from build123d import *

# Parameters (mm, degrees)
EXTRUDE_1_DEPTH     = 38
SKETCH_2_R          = 2.75
CUT_EXTRUDE_1_DEPTH = 21
CUT_EXTRUDE_2_DEPTH = 21


with BuildPart() as part:
    # 草图1 → 凸台-拉伸1 (new body)
    with BuildSketch(Plane(origin=(0, 0, 0), x_dir=(0, 0, -1), z_dir=(1, 0, 0))):
        Polygon((0, 0), (20, 0), (20, 3), (3, 3), (3, 20), (0, 20), align=None)
    extrude(amount=EXTRUDE_1_DEPTH)

    # 草图2 → 切除-拉伸1 (cut, through all)
    with BuildSketch(Plane.XY):
        with Locations((9, 10)):
            Circle(SKETCH_2_R)
        with Locations((29, 10)):
            Circle(SKETCH_2_R)
    extrude(amount=-CUT_EXTRUDE_1_DEPTH, mode=Mode.SUBTRACT)

    # 草图3 → 切除-拉伸2 (cut, through all)
    with BuildSketch(Plane.XZ):
        with BuildLine():
            Line((6.25, -13.5), (6.25, -6.5))
            ThreePointArc((6.25, -6.5), (9, -3.75), (11.75, -6.5))
            Line((11.75, -6.5), (11.75, -13.5))
            ThreePointArc((11.75, -13.5), (9, -16.25), (6.25, -13.5))
        make_face()
        with BuildLine():
            Line((26.25, -13.5), (26.25, -6.5))
            ThreePointArc((26.25, -6.5), (29, -3.75), (31.75, -6.5))
            Line((31.75, -6.5), (31.75, -13.5))
            ThreePointArc((31.75, -13.5), (29, -16.25), (26.25, -13.5))
        make_face()
    extrude(amount=-CUT_EXTRUDE_2_DEPTH, mode=Mode.SUBTRACT)


solid = part.part
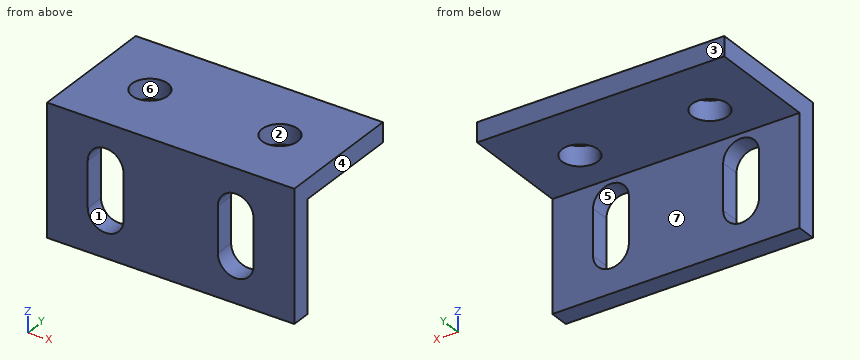
The listing builds one solid part. Answer for the finished solid, in the listing's coordinates (mm). Face numbers are marked on the shaded views. A direction names the side the tool comes from. Give positions to 0.01 mm unless a question says otherwise; leave off trailing zeros. Order: outer loops, then holes, each group sorted by start corner. A loop starts at its lowest first (then second) coordinate and runs counter-clockwise, first axis right, second up. Notation, with made-up numbers: (4, 23) - (42, 23) arc R13 ccw to (42, 43) - close; hole circle Ø7 at (2.5, -3.5). An arc over 180 degrees is marked (long way). Answer as CSV lines item,"result".
Q1. A cutting plane is placed at A-A, the plane y = 10. Determine the outline of the cut face in (x, z).
Answer key:
outline,"(0, -3) - (6.25, -3) - (6.25, 0) - (0, 0) - close; (11.75, -3) - (26.25, -3) - (26.25, 0) - (11.75, 0) - close; (31.75, -3) - (38, -3) - (38, 0) - (31.75, 0) - close"
Q2. Determine the mould class of the marked faces 1, 2, 3 and 4 for opening direction X: pulls with the +X half, pulls with the -X half, needs draft (parallel to the pull), parting line crosses it, or undercut.
Answer key:
face 1,"undercut"
face 2,"undercut"
face 3,"needs draft"
face 4,"pulls with the +X half"
Q3. Each of these flat-tipped pins is pushed along its axis until it touches: pin 1 Ø1 at (x, y) = (28.5, 14.5) entering from -Z; pin 2 Ø10 at (x, z) = (25, -8.5) entering from +Y. Where does it stop, or does it pass through?
Answer key:
pin 1,"stops at z = -3"
pin 2,"stops at y = 3"
Q4. Which of the six approach directions +Z, -Z, +X, -X, +Y, -Y give full straight-line access (tool end or side, diameter ignored) to the marked faces 5, 6 and 7?
Answer key:
face 5,"+Y, -Y"
face 6,"+Z, -Z"
face 7,"-Z, +X, -X, +Y"
Q5. A cutting plane is placed at C-C, the plane z = -5.75. Determine the outline of the cut face in (x, y), and give its area (3 significant figures).
Answer key:
outline,"(0, 0) - (6.35, 0) - (6.35, 3) - (0, 3) - close; (11.65, 0) - (26.35, 0) - (26.35, 3) - (11.65, 3) - close; (31.65, 0) - (38, 0) - (38, 3) - (31.65, 3) - close"
area,"82.3 mm^2"
Q6. A cutting plane is placed at D-D, the plane z = -17.5. Determine the outline of the cut face in (x, y), and give its area (3 significant figures).
Answer key:
outline,"(0, 0) - (38, 0) - (38, 3) - (0, 3) - close"
area,"114 mm^2"
Q7. A cutting plane is placed at B-B, the plane x = 29. Determine the outline of the cut face in (y, z), and give its area (3 significant figures).
Answer key:
outline,"(0, -20) - (3, -20) - (3, -16.25) - (0, -16.25) - close; (0, -3.75) - (3, -3.75) - (3, -3) - (7.25, -3) - (7.25, 0) - (0, 0) - close; (12.75, -3) - (20, -3) - (20, 0) - (12.75, 0) - close"
area,"57.0 mm^2"
Q8. Straight lines are drawn through the part: L1, parallel to Y at x = 9, z = -1.6; L2, parallel to X at y = 2.75, z = -15.25; L3, parallel to Z at x = 6.5, y = 13. For each, find the intervals that lie inside material, in ascending order.
Answer key:
L1,"y = 0 to 7.25, 12.75 to 20"
L2,"x = 0 to 6.88, 11.12 to 26.88, 31.12 to 38"
L3,"z = -3 to 0"
